Source: CAD feature listing. Evaluate the final solid. Frame: model axes, mm. A direction names the side the tool comes from. Round coordinates to 2 decimals unless told otherwise and drop trailing zeros. Write each loop counter-clockwise with the first axis right and the second up, starting at its lowest first coordinate (ties: lowest second). Pieces come first, ordered by that corner, then holes. Notation, with made-up numbers: (-27, -24) -> (3, -24) arc R32 ccw to (3, 12) -> close; hole circle Ø7 at (25.5, 25.25). An arc over 180 degrees is marked (long way). Put each result on its own line as item: value.
```python
from build123d import *

# Parameters (mm, degrees)
F0_R     = 10
F1_DEPTH = 130
F2_R     = 20
F3_DEPTH = 20
F4_R     = 10
F5_R     = 13.239719
F6_DEPTH = 7
F7_R     = 5


with BuildPart() as f1:
    # F0 (on Front) → F1 (new body)
    with BuildSketch(Plane.XZ):
        with Locations((-0.790664, 2.688253)):
            Circle(F0_R)
    extrude(amount=F1_DEPTH)

    # F2 (on face) → F3 (join)
    with BuildSketch(Plane(origin=(0, 0, 0), x_dir=(-1, 0, 0), z_dir=(0, 1, 0))):
        with Locations((0.790664, 2.688253)):
            Circle(F2_R)
    extrude(amount=F3_DEPTH)

    # F4
    f4_edges = [f1.edges().sort_by_distance(p)[0] for p in [
        (19.209336, 20, 2.688253),
    ]]
    fillet(f4_edges, radius=F4_R)

    # F5 (on face) → F6 (join)
    with BuildSketch(Plane.XZ.offset(130)):
        with Locations((-0.790664, 2.688253)):
            Circle(F5_R)
    extrude(amount=-F6_DEPTH)

    # F7
    f7_edges = [f1.edges().sort_by_distance(p)[0] for p in [
        (-14.030383, -130, 2.688253),
    ]]
    fillet(f7_edges, radius=F7_R)


solid = f1.part
```
Q1. Pin query (flat end, axial travel): pin 1 (6 mm diameter, centred on y = -27.5, z = 4, fed in from -X); pin 2 (5 mm diameter, centred on y = -106.5, z = -11.5, fed in from +X); pin 3 (5 mm diameter, centred on x = -5, z = 18.5, fed in from -Y); pin 4 (1 mm diameter, centred on x = -10, y = -107.5, fed in from +Z). Return the tip coordinate at first contact, or that it passes through.
Ans:
pin 1: stops at x = -10.79
pin 2: passes through
pin 3: stops at y = 0
pin 4: stops at z = 7.6
Q2. Draft query along Y for faces 4 (the cylindrical face through (-8.726, -60.639, -3.397)), 5 (the flat face through (-1, -130, 3)), 6 (the cylindrical face through (3.545, 4.93, -16.836)). Return one class per face: +Y half, -Y half, draft (parallel to the pull), parting line (faces both ways), or undercut.
Ans:
face 4: undercut
face 5: -Y half
face 6: draft
Q3. Reachability of faces 1 (the flat face through (-1, 20, 3)), 2 (the flat face through (1, -123, 13)), 3 (the cylindrical face through (11.44, -124.01, -2.38)) from +Z, -Z, +X, -X, +Y, -Y: full face, straight path, thin tool, end or side. Return the list, or none.
Ans:
face 1: +Z, -Z, +X, -X, +Y
face 2: none
face 3: -Y
Q4. Material intervals for line 1 (Y direction, x = -4, z = -7); line 2 (Z direction, x = -1.5, y = -118); line 3 (Y direction, x = 10, z = -8), sorted ascending. Write a range as [from, to].
Ans:
line 1: y = [-129.6, -123], [0, 20]
line 2: z = [-7.29, 12.66]
line 3: y = [0, 18.55]
Q5. Cut plane A-A on y = -98.5. Output: boundary loops of the cut face in (x, z).
Ans:
outline: circle Ø20 at (-0.79, 2.69)
